Model file for the job. Use its own axes, mm. Face numbers are marked on the shaded views. A direction names the side the tool comes from. Round coordinates to 2 decimals unless told otherwise and drop trailing zeros. Loops run counter-clockwise (first coordinate to the right, second up) from the corner with the lowest first, then second, coordinate; pieces in that order, holes last. Notation, with made-up numbers: (31.5, 12.5) - (82.5, 12.5) arc R14 ccw to (82.5, 32.5) - close; hole circle Ø5 at (77, 14.5). An arc over 180 degrees is marked (long way). Use one line per item in the form item = value.
Autodesk Fusion 360 part; units mm, degrees
sketch "Skizze1" plane through (0, 0, 0) normal (0, 0, 1) x (1, 0, 0)
  line L0 (-46.6781, -1) -> (43.3215, -1) construction
  arc A0 (-29.9833, -1) -> (29.9833, -1) centre (0, 0) ccw
  arc A1 (-20.1252, -1) -> (20.1252, -1) centre (0, 0) ccw
  arc A2 (-15.618, -1) -> (15.618, -1) centre (0, 0) ccw
  line L1 (15.618, -1) -> (29.9833, -1)
  line L2 (-15.618, -1) -> (-29.9833, -1)
  point P0 (-29.9833, -1)
  point P1 (-20.1252, -1)
  point P2 (-15.618, -1)
  point P3 (15.618, -1)
  point P4 (20.1252, -1)
  point P5 (29.9833, -1)
  dimension "d6" = 1
  dimension "d7" = 30
  dimension "d8" = 20.15
  dimension "d9" = 15.65
extrude "Extrusion1" add sketch "Skizze1" along normal blind 36
extrude "Extrusion2" cut sketch "Skizze1" along normal blind 5.3 contours A1 A2 L1 L2
sketch "Skizze3" plane through (0, -1, 0) normal (0, 1, 0) x (-1, 0, 0)
  line L0 (20.1252, 5.3) -> (20.1252, 0)
  line L1 (20.1252, 0) -> (29.9833, 0)
  line L2 (29.9833, 0) -> (29.9833, 36)
  line L3 (29.9833, 36) -> (15.618, 36)
  line L4 (15.618, 36) -> (15.618, 5.3)
  line L5 (15.618, 5.3) -> (20.1252, 5.3)
  line L6 (-23, 38.9334) -> (-23, -25) construction
  line L7 (23, 38.9334) -> (23, -33.2487) construction
  line L8 (-52.1355, 10.8) -> (51.6739, 10.8) construction
  line L9 (-50.0712, 25.8) -> (44.4743, 25.8) construction
  circle A0 centre (-23, 25.8) radius 1.75
  circle A1 centre (-23, 10.8) radius 1.75
  circle A2 centre (23, 25.8) radius 1.75
  circle A3 centre (23, 10.8) radius 1.75
  line L10 (-51.02, 5.3) -> (55, 5.3) construction
  line L11 (0, 38.1175) -> (0, -20) construction
  line L12 (-4.5, 5.3) -> (4.5, 5.3)
  line L13 (4.5, 5.3) -> (4.5, -4.7)
  line L14 (4.5, -4.7) -> (-4.5, -4.7)
  line L15 (-4.5, -4.7) -> (-4.5, 5.3)
  arc A4 (4.5, 5.3) -> (-4.5, 5.3) centre (0, 5.3) ccw
  point P0 (-23, 25.8)
  point P1 (-23, 10.8)
  point P2 (23, 25.8)
  point P3 (23, 10.8)
  dimension "d14" = 10.8
  dimension "d15" = 25.8
  dimension "d17" = 3.5
  dimension "d18" = 3.5
  dimension "d19" = 3.5
  dimension "d20" = 3.5
  dimension "d21" = 5.3
  dimension "d29" = 23
  dimension "d30" = 23
extrude "Extrusion3" cut sketch "Skizze3" against normal blind 100 contours A0 | A1 | A2 | A3 | L12 A4 | L12 L13 L14 L15
ref_plane "Arbeitsebene1" through (0, -30, 0) normal (0, 1, 0) x (0, 0, 1)
sketch "Skizze5" plane through (0, -30, 0) normal (0, 1, 0) x (1, 0, 0)
  line L0 (23, -32.4719) -> (23, 19) construction
  line L1 (-23, -30.4738) -> (-23, 19) construction
  line L2 (48, -10.8) -> (-39, -10.8) construction
  line L3 (47, -25.8) -> (-45, -25.8) construction
  circle A0 centre (23, -25.8) radius 5
  circle A1 centre (23, -10.8) radius 5
  circle A2 centre (-23, -25.8) radius 5
  circle A3 centre (-23, -10.8) radius 5
  dimension "d27" = 23
  dimension "d31" = 23
  dimension "d32" = 10.8
  dimension "d33" = 25.8
  dimension "d34" = 10
  dimension "d35" = 10
  dimension "d36" = 10
  dimension "d37" = 10
extrude "Extrusion4" cut sketch "Skizze5" along normal blind 26
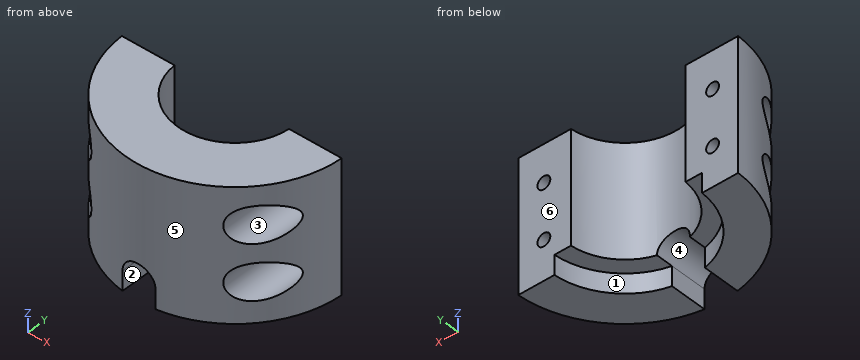
1. Wall check: probe 1 along Z at (x, y) = (-23, -1.85); probe 2 along Z at (x, y) = (-23, -14.5); probe 3 along X at (y, z) = (-9.5, 25.8). Give the ranges that are in metal, low to high.
Geometry check:
probe_1 = 0 to 9.05, 12.55 to 24.05, 27.55 to 36
probe_2 = 0 to 5.8, 15.8 to 20.8, 30.8 to 36
probe_3 = -28.46 to -28, -18 to -12.44, 12.44 to 18, 28 to 28.46
2. Pull direction X, two halves, no side cores. Call the marked faces 4, 5 and 6: +X half, -X half, draft (parallel to the pull), parting line (faces both ways), or undercut.
Geometry check:
face_4 = undercut
face_5 = parting line
face_6 = draft
3. Flat gauge pins, fed straight in: pin 1 (8 mm diameter, centred on x = -14, y = -10, fed in from -Z); pin 2 (5 mm diameter, centred on y = -15.5, z = 24, fed in from -X); pin 3 (2 mm diameter, centred on x = 13, z = 31.5, fed in from +Y); pin 4 (4 mm diameter, centred on y = -24, z = 3.5, fed in from +X). Where does each tip first touch, or does it go through?
Geometry check:
pin_1 = 0
pin_2 = -26.82
pin_3 = -6.99
pin_4 = 20.4
4. Cut at A-A, the plane x = -22. Give the cut face in (y, z).
Geometry check:
outline = (-20.4, 0) - (-1, 0) - (-1, 9.36) - (-4, 9.36) - (-4, 5.9) - (-20.4, 5.9) - close; (-20.4, 15.7) - (-4, 15.7) - (-4, 12.24) - (-1, 12.24) - (-1, 24.36) - (-4, 24.36) - (-4, 20.9) - (-20.4, 20.9) - close; (-20.4, 30.7) - (-4, 30.7) - (-4, 27.24) - (-1, 27.24) - (-1, 36) - (-20.4, 36) - close
5. Cut at D-D, the plane x = 0. Give the cut face in (y, z).
Geometry check:
outline = (-30, 9.8) - (-15.65, 9.8) - (-15.65, 36) - (-30, 36) - close
6. Cut at B-B, the plane z = 10.8. Give the cut face in (x, y), plus the area to 3 significant figures.
Geometry check:
outline = (-29.98, -1) arc R30 ccw to (-28, -10.77) - (-28, -4) - (-24.75, -4) - (-24.75, -1) - close; (-21.25, -4) - (-18, -4) - (-18, -24) arc R30 ccw to (18, -24) - (18, -4) - (21.25, -4) - (21.25, -1) - (15.62, -1) arc R15.65 cw to (-15.62, -1) - (-21.25, -1) - close; (24.75, -4) - (28, -4) - (28, -10.77) arc R30 ccw to (29.98, -1) - (24.75, -1) - close
area = 686 mm^2
7. Cut at C-C, the plane z = 7. Give the cut face in (x, y).
Geometry check:
outline = (-29.98, -1) arc R30 ccw to (-26.25, -14.52) - (-26.25, -4) - (-19.75, -4) - (-19.75, -22.58) arc R30 ccw to (-4.17, -29.71) - (-4.17, -15.09) arc R15.65 cw to (-15.62, -1) - close; (4.17, -29.71) arc R30 ccw to (19.75, -22.58) - (19.75, -4) - (26.25, -4) - (26.25, -14.52) arc R30 ccw to (29.98, -1) - (15.62, -1) arc R15.65 cw to (4.17, -15.09) - close
8. Tool access for the marked faces 1, 2 and 3: list every direction of +Z, -Z, +X, -X, +Y, -Y with a clear straight run to the whole face (end or side of a thin tool).
Geometry check:
face_1 = -Z, +Y
face_2 = -Z, +Y, -Y
face_3 = -Y
